```python
from build123d import *

# Parameters (mm, degrees)
BOSS_EXTRUDE1_DEPTH = 50.8
FILLET1_R           = 25.4
FILLET2_R           = 12.7


with BuildPart() as part:
    # Sketch1 → Boss-Extrude1 (new body)
    with BuildSketch(Plane.XY):
        Polygon((-93.295534025, 241.224648834), (341.304465963, 241.224648834), (341.304465963, -230.262851166), (223.626687979, -230.262851166), (223.626687979, -60.262851166), (24.382243959, -60.262851166), (24.382243959, -230.262851166), (-93.295534025, -230.262851166), align=None)
    extrude(amount=BOSS_EXTRUDE1_DEPTH)

    # Fillet1
    fillet1_edges = [part.edges().sort_by_distance(p)[0] for p in [
        (-93.295534025, 241.224648834, 25.4),
        (341.304465963, 241.224648834, 25.4),
        (341.304465963, -230.262851166, 25.4),
        (223.626687979, -230.262851166, 25.4),
        (223.626687979, -60.262851166, 25.4),
        (24.382243959, -60.262851166, 25.4),
        (24.382243959, -230.262851166, 25.4),
        (-93.295534025, -230.262851166, 25.4),
    ]]
    fillet(fillet1_edges, radius=FILLET1_R)

    # Fillet2
    fillet2_edges = [part.edges().sort_by_distance(p)[0] for p in [
        (24.382243959, -145.262851166, 0),
        (24.382243959, -145.262851166, 50.8),
        (-93.295534025, 5.480898834, 0),
        (124.004465969, 241.224648834, 0),
        (341.304465963, 5.480898834, 0),
        (282.465576971, -230.262851166, 0),
        (223.626687979, -145.262851166, 0),
        (124.004465969, -60.262851166, 0),
        (-34.456645033, -230.262851166, 0),
        (231.066175737, -222.823363409, 0),
        (333.864978205, -222.823363409, 0),
        (333.864978205, 233.785161076, 0),
        (-85.856046267, 233.785161076, 0),
        (-85.856046267, -222.823363409, 0),
        (16.942756201, -222.823363409, 0),
        (-34.456645033, -230.262851166, 50.8),
        (-93.295534025, 5.480898834, 50.8),
        (124.004465969, -60.262851166, 50.8),
        (223.626687979, -145.262851166, 50.8),
        (282.465576971, -230.262851166, 50.8),
        (341.304465963, 5.480898834, 50.8),
        (124.004465969, 241.224648834, 50.8),
        (231.066175737, -222.823363409, 50.8),
        (333.864978205, -222.823363409, 50.8),
        (333.864978205, 233.785161076, 50.8),
        (-85.856046267, 233.785161076, 50.8),
        (-85.856046267, -222.823363409, 50.8),
        (16.942756201, -222.823363409, 50.8),
        (216.187200221, -67.702338924, 0),
        (216.187200221, -67.702338924, 50.8),
        (31.821731717, -67.702338924, 0),
        (31.821731717, -67.702338924, 50.8),
    ]]
    fillet(fillet2_edges, radius=FILLET2_R)


solid = part.part
```
Source: CAD feature listing. Evaluate the final solid. Frame: model axes, mm. A direction names the side the tool comes from. Round coordinates to 2 decimals unless told otherwise and drop trailing zeros. Loops run counter-clockwise (first coordinate to the right, second up) from the corner with the lowest first, then second, coordinate; pieces in that order, holes last. Notation, with made-up numbers: M -38,58 L 4,58 A31 ccw 4,91 Z; hole C 82,-30 d5. An arc over 180 degrees is marked long. Use a Markdown table: item, result. Add a question column.
1. Section query A-A on y = -164. Return the cut outline in (x, z), then the cut area to 3 significant figures.
2. Section query B-B on x = 153. Return the cut outline in (y, z).
3. Section query C-C on z = 21. Return the cut outline in (x, y), then the cut area to 3 significant figures.
4. Contact query for a flat-ended pin moving along its axis: P1, Ø1, axis at x = 57.5, z = 27, coming from the -Y side. Output: stop coordinate, or through.
5. Line query: line 1 (X direction, y = -203, z = 37.5); line 2 (Y direction, x = 136, z = 23); line 3 (Y direction, x = 114, z = 12). Output: solid intervals per line, ascending.
6. Reachability of faces 1 (the cylindrical face through (-34.92, -226.44, 47.18)), 2 (the cylindrical face through (216.38, -67.9, 25.58)), 3 (the cylindrical face through (227.45, -144.43, 3.62)), 4 (the cylindrical face through (122.97, -56.44, 47.18)) from +Z, -Z, +X, -X, +Y, -Y: full face, straight path, thin tool, end or side. Return the list, or none.
Reported:
| question | item | result |
|---|---|---|
| 1 | outline | M -93.3,12.7 A12.7 ccw -80.6,0 L 11.68,0 A12.7 ccw 24.38,12.7 L 24.38,38.1 A12.7 ccw 11.68,50.8 L -80.6,50.8 A12.7 ccw -93.3,38.1 Z; M 223.63,12.7 A12.7 ccw 236.33,0 L 328.6,0 A12.7 ccw 341.3,12.7 L 341.3,38.1 A12.7 ccw 328.6,50.8 L 236.33,50.8 A12.7 ccw 223.63,38.1 Z |
| 1 | area | 11,700 mm² |
| 2 | outline | M -60.26,12.7 A12.7 ccw -47.56,0 L 228.52,0 A12.7 ccw 241.22,12.7 L 241.22,38.1 A12.7 ccw 228.52,50.8 L -47.56,50.8 A12.7 ccw -60.26,38.1 Z |
| 3 | outline | M -93.3,-204.86 A25.4 ccw -67.9,-230.26 L -1.02,-230.26 A25.4 ccw 24.38,-204.86 L 24.38,-85.66 A25.4 cw 49.78,-60.26 L 198.23,-60.26 A25.4 cw 223.63,-85.66 L 223.63,-204.86 A25.4 ccw 249.03,-230.26 L 315.9,-230.26 A25.4 ccw 341.3,-204.86 L 341.3,215.82 A25.4 ccw 315.9,241.22 L -67.9,241.22 A25.4 ccw -93.3,215.82 Z |
| 3 | area | 170,000 mm² |
| 4 | P1 | stops at y = -60.26 |
| 5 | line 1 | x = -93.3 to 24.38, 223.63 to 341.3 |
| 5 | line 2 | y = -60.26 to 241.22 |
| 5 | line 3 | y = -60.24 to 241.21 |
| 6 | face 1 | +Z, +X, -X, -Y |
| 6 | face 2 | +Z, -Z, -Y |
| 6 | face 3 | -Z, -Y |
| 6 | face 4 | +Z, -Y |
